Autodesk Inventor part; units mm, degrees
ref_plane "YZ Plane" through (0, 0, 0) normal (1, 0, 0) x (0, 1, 0)
ref_plane "XZ Plane" through (0, 0, 0) normal (0, 1, 0) x (-1, 0, 0)
ref_plane "XY Plane" through (0, 0, 0) normal (0, 0, 1) x (1, 0, 0)
sketch "Sketch1" plane through (0, 0, 0) normal (0, 0, 1) x (1, 0, 0)
  line L0 (0, 0) -> (15, 0)
  line L1 (15, 0) -> (15, -35)
  line L2 (15, -35) -> (0, -35)
  line L3 (0, -35) -> (0, 0)
  line L4 (0, 0) -> (35, 0)
  line L5 (35, 0) -> (35, -15)
  line L6 (35, -15) -> (0, -15)
  line L7 (0, -15) -> (0, 0)
  dimension "d0" = 15
  dimension "d1" = 35
  dimension "d2" = 35
  dimension "d3" = 15
extrude "Extrusion1" add sketch "Sketch1" along normal blind 25
sketch "Sketch15" plane through (35, -15, 0) normal (1, 0, 0) x (0, 0, -1)
  line L0 (0, 0) -> (-25, 0) construction
  line L1 (0, 0) -> (0, 15) construction
  line L2 (-25, 0) -> (0, 0) construction
  line L3 (0, 0) -> (0, 10.4) construction
  line L4 (0, 10.4) -> (-25, 10.4) construction
  line L5 (-25, 10.4) -> (-25, 0) construction
  line L6 (-20.7, 0) -> (-4.3, 0) construction
  line L7 (-4.3, 0) -> (-4.3, 10.4) construction
  line L8 (-4.3, 10.4) -> (-20.7, 10.4) construction
  line L9 (-20.7, 10.4) -> (-20.7, 0) construction
  line L10 (-20.7, 0) -> (-4.3, 10.4) construction
  line L11 (-4.3, 0) -> (-20.7, 10.4) construction
  circle A0 centre (-15.5, 5.2) radius 5.2
  circle A1 centre (-9.5, 5.2) radius 5.2
  line L12 (-15.5, 0) -> (-9.5, 0)
  line L13 (-9.5, 0) -> (-9.5, 10.4)
  line L14 (-9.5, 10.4) -> (-15.5, 10.4)
  line L15 (-15.5, 10.4) -> (-15.5, 0)
  line L16 (-15.5, 0) -> (-9.5, 10.4) construction
  line L17 (-9.5, 0) -> (-15.5, 10.4) construction
  point P0 (-12.5, 5.2)
  dimension "d58" = 10.4
  dimension "d59" = 16.4
  dimension "d60" = 10.4
extrude "Extrusion9" cut sketch "Sketch15" against normal blind 20
sketch "Sketch16" plane through (0, -35, 0) normal (0, -1, 0) x (1, 0, 0)
  line L0 (15, 25) -> (15, 15.5) construction
  line L1 (35, 0) -> (0, 0) construction
  line L2 (15, 25) -> (4.5, 25) construction
  line L3 (4.5, 25) -> (4.5, 0) construction
  line L4 (4.5, 0) -> (15, 0) construction
  line L5 (15, 0) -> (15, 25) construction
  line L6 (4.5, 20.75) -> (15, 20.75) construction
  line L7 (15, 20.75) -> (15, 4.25) construction
  line L8 (15, 4.25) -> (4.5, 4.25) construction
  line L9 (4.5, 4.25) -> (4.5, 20.75) construction
  line L10 (4.5, 20.75) -> (15, 4.25) construction
  line L11 (15, 20.75) -> (4.5, 4.25) construction
  circle A0 centre (9.75, 15.5) radius 5.25
  circle A1 centre (9.75, 9.5) radius 5.25
  line L12 (15, 15.5) -> (15, 9.5)
  line L13 (4.5, 15.5) -> (15, 15.5)
  line L14 (15, 15.5) -> (15, 9.5)
  line L15 (15, 9.5) -> (4.5, 9.5)
  line L16 (4.5, 9.5) -> (4.5, 15.5)
  line L17 (4.5, 15.5) -> (15, 9.5) construction
  line L18 (15, 15.5) -> (4.5, 9.5) construction
  point P0 (9.75, 12.5)
  dimension "d63" = 10.5
  dimension "d64" = 10.5
  dimension "d65" = 16.5
extrude "Extrusion10" cut sketch "Sketch16" against normal blind 20
fillet "Fillet10" radius 1 6 edges at (4.5, -35, 12.5) (9.75, -35, 4.25) (9.75, -35, 20.75) (35, -4.6, 12.5) (35, -9.8, 4.3) (35, -9.8, 20.7)
fillet "Fillet11" radius 5 1 edges at (0, 0, 12.5)
fillet "Fillet12" radius 3 2 edges at (0, -35, 12.5) (35, 0, 12.5)
properties part number "Gate Corner V5"
Input: part model. Units: mm. Frame: model coordinates. A direction names the side the tool comes from. Coordinates: 2 decimals unless noted, no trailing zeros. Loops run counter-clockwise (first coordinate to the right, second up) from the corner with the lowest first, then second, coordinate; pieces in that order, holes last.
Q1. Set-up query: faces 1 (the flat face through (4.5, -25, 12)), 2 (the flat face through (15, -25, 20)), 3 (the cylindrical face through (34.14, -0.9, 12.68)), 4 (the flat face through (15, -10, 12)), 5 (the flat face through (10, -15, 13)). Return all of +Z, -Z, +X, -X, +Y, -Y with unobstructed straight access to the full face (end or side cutting, diameter ignored); none if empty.
Results are:
face 1: +X, -Y
face 2: +Z, -Z, +X, -Y
face 3: +Z, -Z, +X, +Y
face 4: +X
face 5: -Y
Q2. Section D-D, the plane y = -9.8. Return the cut outline in (x, z).
Results are:
outline: (0, 0) - (35, 0) - (35, 3.3) arc R1 ccw to (34, 4.3) - (15, 4.3) - (15, 20.7) - (34, 20.7) arc R1 ccw to (35, 21.7) - (35, 25) - (0, 25) - close
Q3. Section A-A, the plane y = -22. Return the cut outline in (x, z).
Results are:
outline: (0, 0) - (15, 0) - (15, 9.5) arc R5.25 cw to (4.5, 9.5) - (4.5, 15.5) arc R5.25 cw to (15, 15.5) - (15, 25) - (0, 25) - close
Q4. Contact query for flat-ended pins moving along their axis: pin 1 (10.5 mm diameter, centred on y = -28.5, z = 3, fed in from +X); pin 2 (5 mm diameter, centred on x = 29.5, z = 5, fed in from -Y); pin 3 (3 mm diameter, centred on y = -27, z = 13, fed in from +X). Output: stop coordinate, or through.
Results are:
pin 1: stops at x = 15
pin 2: stops at y = -15
pin 3: stops at x = 4.5
Q5. Section C-C, the plane z = 22.75. Return the cut outline in (x, y), and give its area (3 significant figures).
Results are:
outline: (0, -32) arc R3 ccw to (3, -35) - (15, -35) - (15, -15) - (35, -15) - (35, -3) arc R3 ccw to (32, 0) - (5, 0) arc R5 ccw to (0, -5) - close
area: 816 mm2
Q6. Section B-B, the plane x = 9.75. Return the cut outline in (y, z).
Results are:
outline: (-35, 0) - (0, 0) - (0, 25) - (-35, 25) - (-35, 21.75) arc R1 ccw to (-34, 20.75) - (-15, 20.75) - (-15, 4.25) - (-34, 4.25) arc R1 ccw to (-35, 3.25) - close
Q7. Mould query, pull axis Y, two halves, no side actions, for faces 6 (the cylindrical face through (24.6, -9.7, 20.7)), 7 (the cylindrical face through (24.6, -9.9, 4.3)), 8 (the flat face through (13, -13, 25)), 9 (the flat face through (18, 0, 12)). Classes: +Y half, -Y half, draft (parallel to the pull), parting line (faces both ways), or undercut.
Results are:
face 6: undercut
face 7: undercut
face 8: draft
face 9: +Y half
Q8. Line query: line 1 along Z through (x, y) = (10, -24); line 2 along X through (y, z) = (-8.5, 12.5); line 3 along Y through (x, z) = (18.5, 3.25). Output: solid intervals per line, ascending.
Results are:
line 1: z = 0 to 4.26, 20.74 to 25
line 2: x = 0 to 15
line 3: y = -15 to 0
